```python
from build123d import *

# Parameters (mm, degrees)
CUT_EXTRUDE_1_DEPTH         = 43.576377572
HOLE_WIZARD_10_0_10_1_D     = 10
HOLE_WIZARD_10_0_10_1_DEPTH = 16.995696905
HOLE_WIZARD_10_0_10_1_TIP   = 3.004303095
FILLET_1_R                  = 1


with BuildPart() as part:
    # 草图1 → 旋转1 (revolve)
    with BuildSketch(Plane.XY, mode=Mode.PRIVATE) as revolve_1_sk:
        with BuildLine():
            Line((0, 0), (-14, 0))
            Line((-14, 0), (-14, 16.165246825))
            Line((-14, 16.165246825), (-27, 16.165246825))
            Line((-27, 16.165246825), (-27, 32.165246825))
            ThreePointArc((-27, 32.165246825), (-13.574201869, 34.289369415), (0, 35))
            Line((0, 35), (0, 0))
        make_face()
    revolve(revolve_1_sk.sketch.rotate(Axis((0, 0, 0), (0, 1, 0)), 270), axis=Axis((0, 0, 0), (0, 1, 0)))

    # 草图2 → 切除-拉伸1 (cut, through all)
    with BuildSketch(Plane.XZ.offset(-16.165246825)):
        with BuildLine():
            ThreePointArc((-26.636693093, 4.414360778), (-19.378362398, 11.188102747), (-17.141295122, 20.860872502))
            ThreePointArc((-17.141295122, 20.860872502), (-23.382685902, 13.5), (-26.636693093, 4.414360778))
        make_face()
        with BuildLine():
            ThreePointArc((9.495397971, 25.27523328), (0, 27), (-9.495397971, 25.27523328))
            ThreePointArc((-9.495397971, 25.27523328), (0, 22.376205494), (9.495397971, 25.27523328))
        make_face()
        with BuildLine():
            ThreePointArc((26.636693093, 4.414360778), (23.382685902, 13.5), (17.141295122, 20.860872502))
            ThreePointArc((17.141295122, 20.860872502), (19.378362398, 11.188102747), (26.636693093, 4.414360778))
        make_face()
        with BuildLine():
            ThreePointArc((17.141295122, -20.860872502), (23.382685902, -13.5), (26.636693093, -4.414360778))
            ThreePointArc((26.636693093, -4.414360778), (19.378362398, -11.188102747), (17.141295122, -20.860872502))
        make_face()
        with BuildLine():
            ThreePointArc((9.495397971, -25.27523328), (0, -22.376205494), (-9.495397971, -25.27523328))
            ThreePointArc((-9.495397971, -25.27523328), (0, -27), (9.495397971, -25.27523328))
        make_face()
        with BuildLine():
            ThreePointArc((-17.141295122, -20.860872502), (-19.378362398, -11.188102747), (-26.636693093, -4.414360778))
            ThreePointArc((-26.636693093, -4.414360778), (-23.382685902, -13.5), (-17.141295122, -20.860872502))
        make_face()
    extrude(amount=-CUT_EXTRUDE_1_DEPTH, mode=Mode.SUBTRACT)

    # Ø10.0 (10) 直径孔1
    with Locations(Plane(origin=(0, 0, 0), x_dir=(-1, 0, 0), z_dir=(0, -1, 0))):
        with Locations((0, 0)):
            Hole(HOLE_WIZARD_10_0_10_1_D / 2, depth=HOLE_WIZARD_10_0_10_1_DEPTH)
            with Locations((0, 0, -(HOLE_WIZARD_10_0_10_1_DEPTH + HOLE_WIZARD_10_0_10_1_TIP / 2))):  # 118° drill point
                Cone(0, HOLE_WIZARD_10_0_10_1_D / 2, HOLE_WIZARD_10_0_10_1_TIP, mode=Mode.SUBTRACT)

    # 圆角1
    fillet_1_edges = [part.edges().sort_by_distance(p)[0] for p in [
        (0, 0, 14),
    ]]
    fillet(fillet_1_edges, radius=FILLET_1_R)


solid = part.part
```
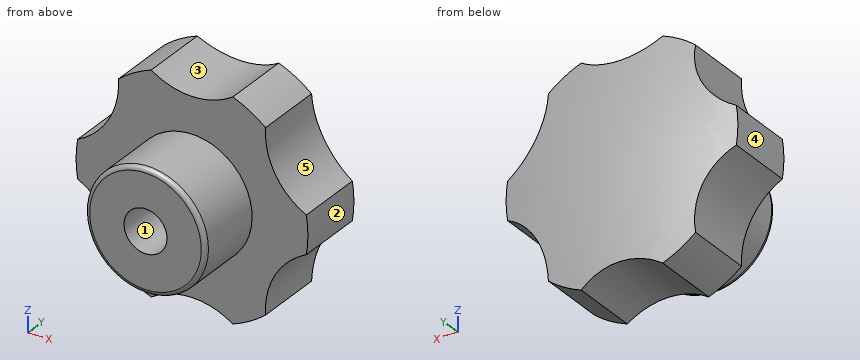
Design review of the part built by this model. Coordinates are the model's own, in mm. Face numbers are marked on the shaded views. A direction names the side the tool comes from. Round coordinates to 2 decimals unless told otherwise and drop trailing zeros. Write each loop counter-clockwise with the first axis right and the second up, starting at its lowest first coordinate (ties: lowest second). Pieces come first, ordered by that corner, then holes. Notation, with made-up numbers: (-14.75, -11.5) -> (16.25, -11.5) arc R21 cw to (16.25, -4.5) -> close; hole circle Ø9 at (78, 75). An arc over 180 degrees is marked (long way). Answer in a Markdown table with one row per item.
Q1. Take a section at A-A, the plane y = 29. State the section outline as (x, z) points.
The answers:
| item | result |
|---|---|
| outline | (-26.64, -4.41) arc R17 cw to (-17.14, -20.86) arc R27 ccw to (-9.5, -25.28) arc R17 cw to (9.5, -25.28) arc R27 ccw to (17.14, -20.86) arc R17 cw to (26.64, -4.41) arc R27 ccw to (26.64, 4.41) arc R17 cw to (17.14, 20.86) arc R27 ccw to (9.5, 25.28) arc R17 cw to (-9.5, 25.28) arc R27 ccw to (-17.14, 20.86) arc R17 cw to (-26.64, 4.41) arc R27 ccw to start |
Q2. Clearance check with flat-ended pins moving along their axes: pin 1 Ø4 at (x, z) = (-15, 14) entering from +Y; pin 2 Ø6 at (y, z) = (27, -1) entering from +X; pin 3 Ø6 at (x, z) = (0, 0) entering from -Y. State where each tip first meets the part, or that it passes through.
The answers:
| item | result |
|---|---|
| pin 1 | y = 33.67 |
| pin 2 | x = 27 |
| pin 3 | y = 18.2 |
Q3. Take a section at B-B, the plane y = 15. State the section outline as (x, z) points, then the cut area to 3 significant figures.
The answers:
| item | result |
|---|---|
| outline | circle Ø28 at (0, 0); hole circle Ø10 at (0, 0) |
| area | 537 mm² |
Q4. For the marked faces 1 and 2, list the 3-axis set-ups (+Z, -Z, +X, -X, +Y, -Y) from which the entire face can be reached by the end or side of a thin tool; tool diameter is ignored.
The answers:
| item | result |
|---|---|
| face 1 | -Y |
| face 2 | +X, +Y, -Y |
Q5. Draft analysis for pull direction X (two halves, no side actions). For the marked faces 3, 4 and 5, state which applies: +X half, -X half, draft (parallel to the pull), parting line (faces both ways), or undercut.
The answers:
| item | result |
|---|---|
| face 3 | undercut |
| face 4 | -X half |
| face 5 | +X half |
Q6. Take a section at D-D, the plane z = 15. State the section outline as (x, y) points.
The answers:
| item | result |
|---|---|
| outline | (-17.76, 16.17) -> (17.76, 16.17) -> (17.76, 32.9) arc R129.13 ccw to (-17.76, 32.9) -> close |
Q7. To check wall thickness, follow L1, parallel to X at y = 14, z = 10.5; L2, parallel to Z at x = 15, y = 28; L3, parallel to Y at x = 0.5, z = -1. State the ranges of each line that lie inside material, in increasing order. Write a range as [from, to].
The answers:
| item | result |
|---|---|
| L1 | [-9.26, 9.26] |
| L2 | [-22.45, 22.45] |
| L3 | [19.33, 35] |
Q8. Take a section at C-C, the plane x = -20. State the section outline as (y, z) points, then the cut area to 3 significant figures.
The answers:
| item | result |
|---|---|
| outline | (16.17, -10.19) -> (33.05, -10.19) arc R128.45 ccw to (33.05, 10.19) -> (16.17, 10.19) -> close |
| area | 350 mm² |
